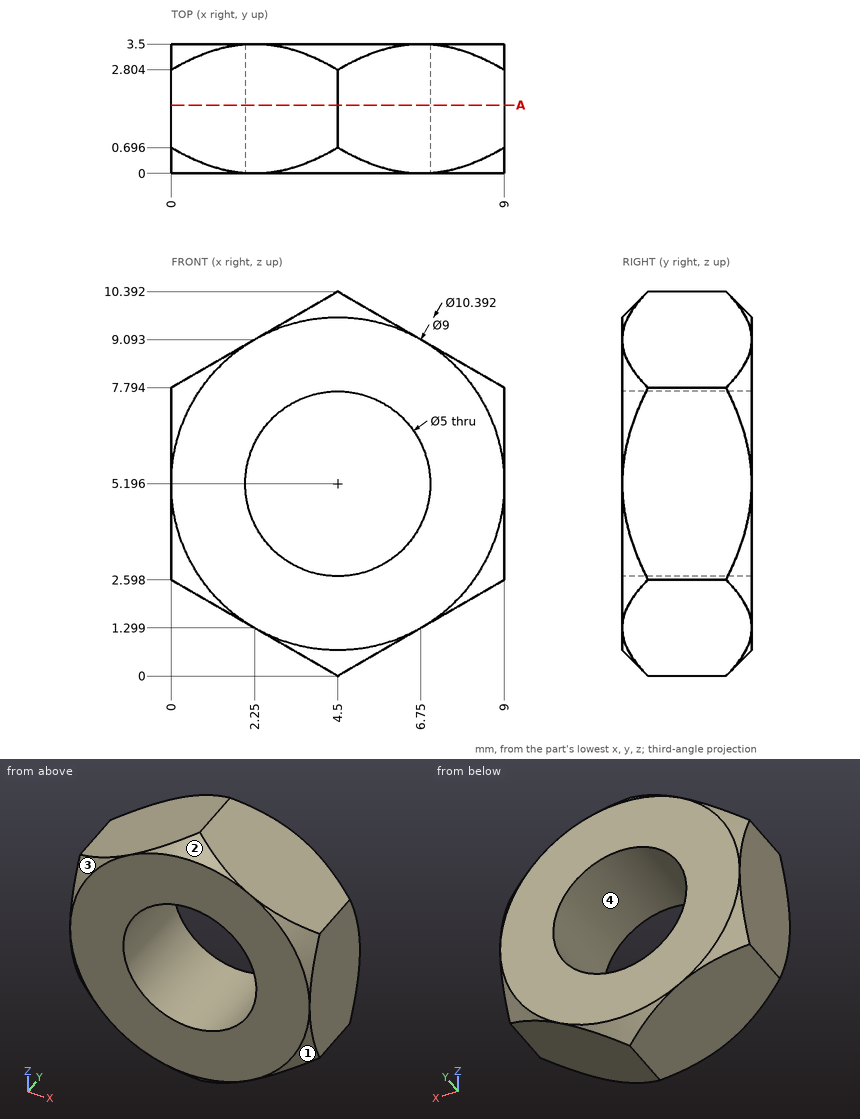
Input: dimensioned drawing with shaded views. Units: mm. Origin: part minimum x, y, z. Coordinates: 2 decimals unless noted, no trailing zeros. Order: outer loops, then holes, each group sorted by start corner. A loop starts at its lowest first (then second) coordinate and runs counter-clockwise, first axis right, second up.
Item 1: Draft query along X for the marked faces 1, 2, 3 and 4. Return one class per face: released by +X, released by -X, zero draft, split by the parting line, or undercut.
Answer:
face 1: released by +X
face 2: split by the parting line
face 3: released by -X
face 4: undercut
Item 2: Contact query for flat-ended pins moving along their axis: P1, Ø1.5, axis at x = 6, y = 1, coming from the +Z side; P2, Ø2, axis at x = 3, y = 2.5, coming from the -Z side. Output: stop coordinate, or through.
Answer:
P1: stops at z = 9.96
P2: stops at z = 0.29
Item 3: Material intervals for line 1 along Z through (x, y) = (6.5, 2.65) (1 decimal); line 2 along X through (y, z) = (1, 7.5); line 3 along X through (y, z) = (3.3, 7), sorted ascending.
Answer:
line 1: z = 1.2 to 3.7, 6.7 to 9.2
line 2: x = 0 to 3.53, 5.47 to 9
line 3: x = 0.16 to 2.77, 6.23 to 8.84
Item 4: Section query A-A (y = 1.85). Output: boundary loops of the cut face in (x, z).
Answer:
outline: (0, 2.6) - (4.5, 0) - (9, 2.6) - (9, 7.79) - (4.5, 10.39) - (0, 7.79) - close; hole circle Ø5 at (4.5, 5.2)
